Geometry: final body of the model. Coordinates: model frame, mm. Face numbers are marked on the shaded views. A direction names the side the tool comes from. Round coordinates to 2 decimals unless told otherwise and drop trailing zeros. Write each loop counter-clockwise with the first axis right and the second up, starting at its lowest first coordinate (ties: lowest second). Pieces come first, ordered by that corner, then holes. Notation, with made-up numbers: M 17,-25.5 L 75,-25.5 A15 cw 75,-17.5 Z; hole C 58.25,-32.5 d9. An arc over 180 degrees is marked long. Use one line per item in the form item = value. Start each with the question number.
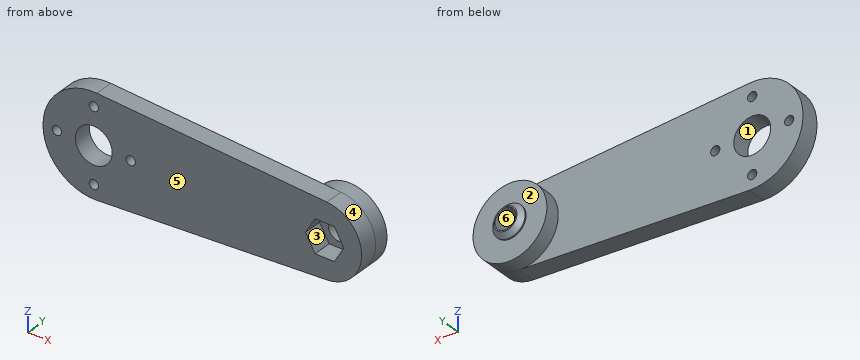
Autodesk Inventor part; units mm, degrees
ref_plane "YZ Plane" through (0, 0, 0) normal (1, 0, 0) x (0, 1, 0)
ref_plane "XZ Plane" through (0, 0, 0) normal (0, 1, 0) x (-1, 0, 0)
ref_plane "XY Plane" through (0, 0, 0) normal (0, 0, 1) x (1, 0, 0)
sketch "Эскиз1" plane through (0, 0, 0) normal (0, 1, 0) x (-1, 0, 0)
  arc A0 (-0.66, -10.9802) -> (-0.66, 10.9802) centre (0, 0) ccw
  line L0 (0, 0) -> (-50, 0) construction
  arc A1 (-50.48, 7.9856) -> (-50.48, -7.9856) centre (-50, 0) ccw
  circle A2 centre (-50, 0) radius 2.25
  circle A3 centre (0, 0) radius 4
  line L1 (-0.66, 10.9802) -> (-50.48, 7.9856)
  line L2 (-50.48, -7.9856) -> (-0.66, -10.9802)
  line L3 (0, 14.7919) -> (0, -15.3295) construction
  circle A4 centre (0, 8) radius 1
  circle A5 centre (-8, 0) radius 1
  circle A6 centre (0, -8) radius 1
  circle A7 centre (8, 0) radius 1
  dimension "d0" = 22
  dimension "d1" = 16
  dimension "d2" = 4.5
  dimension "d3" = 8
  dimension "d4" = 50
  dimension "d7" = 2
  dimension "d8" = 8
  dimension "d25" = 360
extrude "Выдавливание1" add sketch "Эскиз1" along normal blind 4
sketch "Эскиз3" plane through (0, 0, 0) normal (0, -1, 0) x (1, 0, 0)
  circle A0 centre (50, 0) radius 2.25
  circle A1 centre (50, 0) radius 8
  arc A2 (50.48, -7.9856) -> (50.48, 7.9856) centre (50, 0) ccw
  point P0 (0, 0)
extrude "Выдавливание3" add sketch "Эскиз3" against normal blind 7.25
sketch "Эскиз5" plane through (0, 4, 0) normal (0, 1, 0) x (1, 0, 0)
  circle A0 centre (50, 0) radius 2.25
  line L0 (54.1569, 0) -> (52.0785, -3.6)
  line L1 (52.0785, -3.6) -> (47.9215, -3.6)
  line L2 (47.9215, -3.6) -> (45.8431, 0)
  line L3 (45.8431, 0) -> (47.9215, 3.6)
  line L4 (47.9215, 3.6) -> (52.0785, 3.6)
  line L5 (52.0785, 3.6) -> (54.1569, 0)
  point P0 (0, 0)
  dimension "d20" = 7.2
  dimension "d31" = 4.1569
  dimension "d32" = 3.6
  dimension "d33" = 50
extrude "Выдавливание8" cut sketch "Эскиз5" against normal blind 4
sketch "Эскиз8" plane through (50, 7.25, 0) normal (0, 1, 0) x (1, 0, 0)
  circle A0 centre (0, 0) radius 2.25
  circle A1 centre (0, 0) radius 2.2361
  circle A2 centre (0, 0) radius 3.5
  point P0 (-50, 0)
  dimension "d38" = 7
extrude "Выдавливание9" add sketch "Эскиз8" along normal blind 1.3 contours A2
chamfer "Фаска2" distance 1 angle 45 1 edges at (46.5, 8.55, 0)
properties part number "04-01-Качалка"
1. Pull-direction query (Z, two-part tool) for the marked faces 4, 5 and 6; classes: released by +Z, released by -Z, zero draft, split by the parting line, or undercut.
2. Section query C-C (x = 8). Return loops of the section in (y, z).
3. Contact query for flat-ended pins moving along their axis: pin 1 (1.2 mm diameter, centred on x = -8, z = 0, fed in from +Y); pin 2 (3 mm diameter, centred on x = 23.5, y = 2, fed in from +Z); pin 3 (10.5 mm diameter, centred on x = 0, z = 0, fed in from +Y); pin 4 (5 mm diameter, centred on x = 50, z = 0, fed in from -Y). Output: stop coordinate, or through.
4. Section query A-A (x = 0). Return loops of the section in (y, z).
5. Section query D-D (z = 5). Return loops of the section in (x, y) (3 decimals).
6. Ray query, probe 1 along Z at (x, y) = (0, 2); probe 2 along Y at (x, z) = (27, -5); probe 3 along X at (y, z) = (1.75, -3). Return the intervals inside material, ascending.
7. Set-up query: the marked faces 1, 2 and 3. Return all of +Z, -Z, +X, -X, +Y, -Y with unobstructed straight access to the full face (end or side cutting, diameter ignored); none if empty.
8. Section query B-B (y = 2.5). Return loops of the section in (x, z), then the cut area to 3 significant figures.
Checks:
q1.face_4 = split by the parting line
q1.face_5 = zero draft
q1.face_6 = undercut
q2.outline = M 0,-10.54 L 4,-10.54 L 4,-1 L 0,-1 Z; M 0,1 L 4,1 L 4,10.54 L 0,10.54 Z
q3.pin_1 = through
q3.pin_2 = 9.7
q3.pin_3 = 4
q3.pin_4 = 4
q4.outline = M 0,-11 L 4,-11 L 4,-9 L 0,-9 Z; M 0,-7 L 4,-7 L 4,-4 L 0,-4 Z; M 0,4 L 4,4 L 4,7 L 0,7 Z; M 0,9 L 4,9 L 4,11 L 0,11 Z
q5.outline = M -9.798,0 L 56.245,0 L 56.245,7.25 L 43.755,7.25 L 43.755,4 L -9.798,4 Z
q6.probe_1 = -11 to -9, -7 to -4, 4 to 7, 9 to 11
q6.probe_2 = 0 to 4
q6.probe_3 = -10.58 to -2.65, 2.65 to 47.58, 52.42 to 57.42
q7.face_1 = +Y, -Y
q7.face_2 = +Y
q7.face_3 = -Y
q8.outline = M 0.66,-10.98 L 50.48,-7.99 A8 ccw 50.48,7.99 L 0.66,10.98 A11 ccw long Z; hole C -8,0 d2; hole C 0,0 d8; hole C 0,-8 d2; hole C 0,8 d2; hole C 8,0 d2; hole M 45.84,0 L 47.92,-3.6 L 52.08,-3.6 L 54.16,0 L 52.08,3.6 L 47.92,3.6 Z
q8.area = 1,130 mm^2
